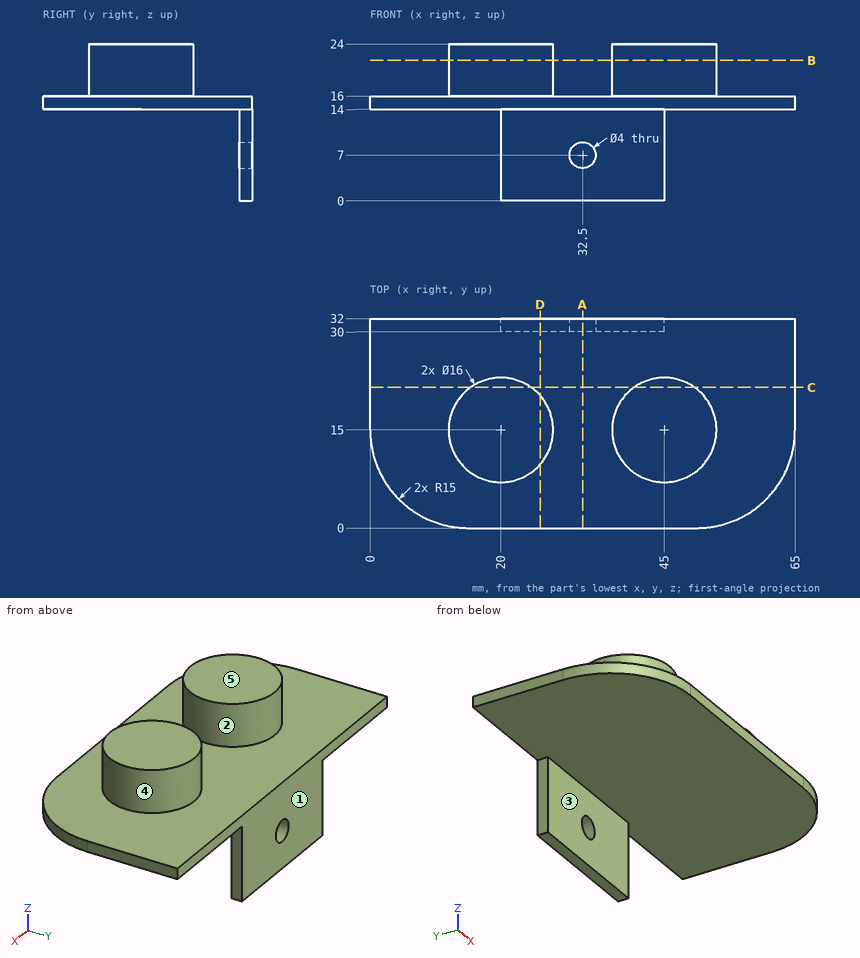
Check sheet for the drawn part. Datum: minimum x, y, z corner. Units: mm. A direction names the side the tool comes from. Give positions to 0.01 mm unless a question says otherwise; leave off trailing zeros. Write each loop counter-clockwise with the first axis right and the second up, starting at its lowest first coordinate (ties: lowest second). Pieces come first, ordered by that corner, then holes.
(1) Cross-section at C-C (y = 21.5). Enter the section's corners in (x, z), plus the area to 3 significant figures.
(2) Cross-section at A-A (x = 32.5). Enter the section's corners in (y, z), plus the area to 3 significant figures.
(3) Gauge pin test, flat ends, axial feed: pin 1 (2 mm diameter, centred on y = 31, z = 10, fed in from -X); pin 2 (6 mm diameter, centred on x = 22.5, y = 20.5, fed in from -Z); pin 3 (2 mm diameter, centred on y = 7.5, z = 17.5, fed in from -X). Record the tip position at first contact, or that the pin passes through.
(4) Cross-section at B-B (z = 21.5). Enter the section's corners in (x, y), plus the area to 3 significant figures.
(5) Access from +Z, -Z, +X, -X, +Y, -Y to the whole of each face (thin tool, end or side, straight path). Record for the marked faces 1, 2 and 3.
(6) Cross-section at D-D (x = 26). Enter the section's corners in (y, z), plus the area to 3 significant figures.
(7) Material ranges on line 1 (Z direction, x = 32.5, y = 31); line 2 (X direction, y = 30.6, z = 7); line 3 (Z direction, x = 14, y = 9), recorded low to high.
(8) Mould release check, pull along X, two halves, no side actions. Record for the marked faces 4 and 5: +X half, -X half, draft (parallel to the pull), parting line (faces both ways), or undercut.
Worked out:
1. outline: (0, 14) - (65, 14) - (65, 16) - (49.66, 16) - (49.66, 24) - (40.34, 24) - (40.34, 16) - (24.66, 16) - (24.66, 24) - (15.34, 24) - (15.34, 16) - (0, 16) - close
1. area: 279 mm2
2. outline: (0, 14) - (30, 14) - (30, 9) - (32, 9) - (32, 16) - (0, 16) - close; (30, 0) - (32, 0) - (32, 5) - (30, 5) - close
2. area: 84.0 mm2
3. pin 1: stops at x = 20
3. pin 2: stops at z = 14
3. pin 3: stops at x = 15.34
4. outline: circle Ø16 at (20, 15); circle Ø16 at (45, 15)
4. area: 402 mm2
5. face 1: +Z, -Z, +X, -X, +Y
5. face 2: +Z
5. face 3: -Z, +X, -X, -Y
6. outline: (0, 14) - (30, 14) - (30, 0) - (32, 0) - (32, 16) - (20.29, 16) - (20.29, 24) - (9.71, 24) - (9.71, 16) - (0, 16) - close
6. area: 177 mm2
7. line 1: z = 0 to 5, 9 to 16
7. line 2: x = 20 to 30.5, 34.5 to 45
7. line 3: z = 14 to 16
8. face 4: undercut
8. face 5: draft
